Autodesk Inventor part; units mm, degrees
ref_plane "YZ Plane" through (0, 0, 0) normal (1, 0, 0) x (0, 1, 0)
ref_plane "XZ Plane" through (0, 0, 0) normal (0, 1, 0) x (-1, 0, 0)
ref_plane "XY Plane" through (0, 0, 0) normal (0, 0, 1) x (1, 0, 0)
sketch "Sketch1" plane through (0, 0, 0) normal (0, 0, 1) x (1, 0, 0)
  line L0 (-19.557, 9.6136) -> (20.443, 9.6136)
  line L1 (20.443, 9.6136) -> (20.443, -10.3864)
  line L2 (20.443, -10.3864) -> (-19.557, -10.3864)
  line L3 (-19.557, -10.3864) -> (-19.557, 9.6136)
  point P0 (0, 0)
  dimension "d0" = 40
  dimension "d1" = 20
extrude "Extrusion1" add sketch "Sketch1" along normal blind 37
sketch "Sketch2" plane through (0, 0, 37) normal (0, 0, 1) x (1, 0, 0)
  line L0 (20.443, 9.6136) -> (20.443, -10.3864)
  line L1 (-19.557, 9.6136) -> (20.443, 9.6136)
  line L2 (-19.557, -10.3864) -> (-19.557, 9.6136)
  line L3 (20.443, -10.3864) -> (-19.557, -10.3864)
  line L4 (-14.557, 8.4886) -> (12.443, 8.4886)
  line L5 (12.443, -9.2614) -> (-14.557, -9.2614)
  line L6 (-14.557, -9.2614) -> (-14.557, 8.4886)
  arc A0 (12.443, -9.2614) -> (12.443, 8.4886) centre (10.3169, -0.3864) ccw
  arc A1 (-14.557, 3.1386) -> (-14.557, -3.9114) centre (-11.6119, -0.3864) ccw
  point P0 (0, 0)
  dimension "d6" = 5
  dimension "d8" = 27
  dimension "d9" = 27
  dimension "d10" = 5.35
  dimension "d11" = 5.35
extrude "Extrusion2" cut sketch "Sketch2" against normal blind 3.15
sketch "Sketch3" plane through (20.443, -10.3864, 0) normal (1, 0, 0) x (0, 0, -1)
  line L0 (-33.85, 20) -> (-33.85, 0)
  line L1 (0, 0) -> (-33.85, 0)
  line L2 (0, 20) -> (0, 0)
  line L3 (0, 20) -> (-33.85, 20)
  point P0 (0, 10.3864)
sketch "Sketch4" plane through (20.443, -10.3864, 0) normal (1, 0, 0) x (0, 0, -1)
  line L0 (-33.85, 20) -> (-33.85, 0)
  line L1 (0, 0) -> (-33.85, 0)
  line L2 (0, 20) -> (-33.85, 20)
  line L3 (-30, 20) -> (-26.85, 20)
  line L4 (-26.85, 20) -> (-26.85, 0)
  line L5 (-26.85, 0) -> (-30, 0)
  line L6 (-30, 0) -> (-30, 20)
  line L7 (-33.85, 0) -> (-33.85, 20)
  line L8 (0, 20) -> (-33.85, 20)
  line L9 (0, 0) -> (0, 20)
  line L10 (0, 0) -> (-33.85, 0)
  point P0 (0, 10.3864)
  dimension "d14" = 7
  dimension "d15" = 3.15
extrude "Extrusion3" add sketch "Sketch4" along normal blind 6.5 contours L2 L4 L1 L6
sketch "Sketch5" plane through (-19.557, -10.3864, 0) normal (-1, 0, 0) x (0, 0, 1)
  line L0 (33.85, 0) -> (33.85, 20)
  line L1 (0, 20) -> (33.85, 20)
  line L2 (0, 0) -> (33.85, 0)
  line L3 (26.85, 0) -> (30, 0)
  line L4 (30, 0) -> (30, 20)
  line L5 (30, 20) -> (26.85, 20)
  line L6 (26.85, 20) -> (26.85, 0)
  point P0 (0, 10.3864)
  dimension "d18" = 7
  dimension "d19" = 3.15
extrude "Extrusion4" add sketch "Sketch5" along normal blind 6.5 contours L2 L6 L1 L4
sketch "Sketch6" plane through (0, 0, 37) normal (0, 0, 1) x (1, 0, 0)
  circle A0 centre (11.193, -0.3864) radius 5.318
  line L0 (20.443, 9.6136) -> (20.443, -10.3864)
  circle A1 centre (11.193, -0.3864) radius 2.5
  point P0 (0, 0)
  dimension "d22" = 9.25
  dimension "d42" = 10.6361
  dimension "d75" = 5
sketch "Sketch7" plane through (20.443, -10.3864, 30) normal (0, 0, 1) x (1, 0, 0)
  line L0 (6.5, 0) -> (6.5, 20)
  line L1 (0, 20) -> (6.5, 20)
  circle A0 centre (4, 5) radius 2.5
  circle A1 centre (4, 15) radius 2.5
  line L2 (0, 0) -> (0, 20)
  point P0 (-20.443, 10.3864)
  point P1 (5.6248, 3.1)
  point P2 (6.5, 3.3)
  point P3 (6.0702, 6.4015)
  point P4 (6.5, 6.3)
  point P5 (6, 13.5)
  point P6 (6.5, 13.7)
  point P7 (6, 16.5)
  point P8 (6.5, 16.7)
  dimension "d25" = 5
  dimension "d26" = 5
  dimension "d79" = 10
  dimension "d80" = 5
  dimension "d81" = 4
  dimension "d82" = 4
sketch "Sketch8" plane through (-19.557, -10.3864, 30) normal (0, 0, 1) x (1, 0, 0)
  line L0 (-7.5004, 19.9995) -> (-7.5004, -0.0005)
  line L1 (-0.5, -0.0005) -> (-7.5004, -0.0005)
  line L2 (-0.4577, 19.9995) -> (-7.5004, 19.9995)
  circle A0 centre (-4, 14.9995) radius 2.5
  circle A1 centre (-4, 4.9995) radius 2.5
  line L3 (0, 20) -> (0, 0)
  point P0 (19.557, 10.3864)
  point P1 (-20.443, 10.3864)
  point P2 (-6, 16.4995)
  point P3 (-7.5004, 16.6995)
  point P4 (-6, 13.4995)
  point P5 (-7.5004, 13.6995)
  point P6 (-6, 6.4995)
  point P7 (-7.5004, 6.2995)
  point P8 (-6, 3.4995)
  point P9 (-7.5004, 3.2995)
  dimension "d35" = 5
  dimension "d36" = 5
  dimension "d37" = 5
  dimension "d38" = 5
  dimension "d83" = 10
  dimension "d84" = 4
  dimension "d85" = 4
extrude "Extrusion7" add sketch "Sketch6" along normal blind 2 contours A0 | A1
hole "Hole1" at (24.443, 4.6136, 30) at (24.443, -5.3864, 30) direction (0, 0, -1) diameter 3 end through all
hole "Hole2" at (-23.557, 4.6131, 30) at (-23.557, -5.3869, 30) direction (0, 0, -1) diameter 3 end through all
extrude "Extrusion14" add sketch "Sketch6" along normal blind 5 contours A1
properties part number "servo HS-7955GT"
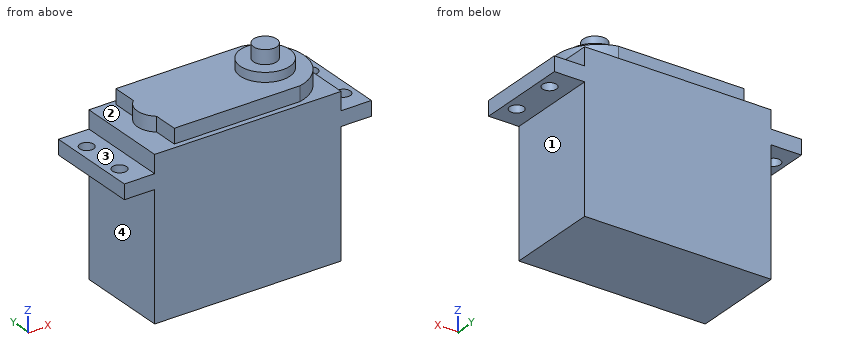
Geometry check sheet. Reference: the model listing, model coordinates, mm. Face numbers are marked on the shaded views. A direction names the side the tool comes from. Give positions to 0.01 mm unless a question says otherwise; leave off trailing zeros. Write each loop counter-clockwise with the first axis right and the second up, starting at its lowest first coordinate (ties: lowest second). Pieces come first, ordered by that corner, then holes. Notation, with made-up numbers: (-7.5, 54.25) - (48.5, 54.25) arc R28 cw to (48.5, 88.25) - close; hole circle Ø9 at (-8.5, 40.25). An arc over 180 degrees is marked (long way). Use a Markdown table: item, result.
Q1. Thickness scan on L1, parallel to Z at x = -13, y = -4.5; L2, parallel to Z at x = -19.5, y = -8.25; L3, parallel to X at y = -6.75, z = 23.5. Record the ranges inside material, lowest first. Write a range as [from, to].
Computed:
| item | result |
|---|---|
| L1 | z = [0, 37] |
| L2 | z = [0, 33.85] |
| L3 | x = [-19.56, 20.44] |
Q2. Set-up check for the marked faces 1, 2, 3 and 4: record each of +Z, -Z, +X, -X, +Y, -Y from which the full face is reachable in a straight line by a thin tool's end or side.
Computed:
| item | result |
|---|---|
| face 1 | -Z, +X, +Y, -Y |
| face 2 | +Z |
| face 3 | +Z, -X, +Y, -Y |
| face 4 | -Z, -X, +Y, -Y |
Q3. Section check D-D, the plane x = 8. Enter the section's corners in (y, z).
Computed:
| item | result |
|---|---|
| outline | (-10.39, 0) - (9.61, 0) - (9.61, 33.85) - (8.49, 33.85) - (8.49, 37) - (3.87, 37) - (3.87, 39) - (-4.64, 39) - (-4.64, 37) - (-9.26, 37) - (-9.26, 33.85) - (-10.39, 33.85) - close |
Q4. Section check B-B, the plane y = -7.5. Enter the section's corners in (x, z), then the cut area to 3 significant figures.
Computed:
| item | result |
|---|---|
| outline | (-26.06, 26.85) - (-19.56, 26.85) - (-19.56, 0) - (20.44, 0) - (20.44, 26.85) - (26.94, 26.85) - (26.94, 30) - (20.44, 30) - (20.44, 33.85) - (16.03, 33.85) - (16.03, 37) - (-14.56, 37) - (-14.56, 33.85) - (-19.56, 33.85) - (-19.56, 30) - (-26.06, 30) - close |
| area | 1,490 mm² |
Q5. Section check C-C, the plane z = 3. Enter the section's corners in (x, y).
Computed:
| item | result |
|---|---|
| outline | (-19.56, -10.39) - (20.44, -10.39) - (20.44, 9.61) - (-19.56, 9.61) - close |
Q6. Section check A-A, the plane x = -9. Enter the section's corners in (y, z), then the cut area to 3 significant figures.
Computed:
| item | result |
|---|---|
| outline | (-10.39, 0) - (9.61, 0) - (9.61, 33.85) - (8.49, 33.85) - (8.49, 37) - (-9.26, 37) - (-9.26, 33.85) - (-10.39, 33.85) - close |
| area | 733 mm² |
Q7. Go/stop test with flat-tipped pins: P1, Ø10, axis at y = -5.5, z = 8, coming from the -X side; P2, Ø8, axis at y = 1.5, z = 12.5, coming from the +X side; P3, Ø3, axis at x = -23.5, y = 4, coming from the +Z side; P4, Ø2.5, axis at x = -23.56, y = 4.61, coming from the +Z side. Record where each tip stops, or that it passes through.
Computed:
| item | result |
|---|---|
| P1 | stops at x = -19.56 |
| P2 | stops at x = 20.44 |
| P3 | stops at z = 30 |
| P4 | passes through |
